Here's how the part is built. I have some questions about the finished solid (model axes, mm). A direction names the side the tool comes from. Round coordinates to 2 decimals unless told otherwise and drop trailing zeros. Write each loop counter-clockwise with the first axis right and the second up, starting at its lowest first coordinate (ties: lowest second). Pieces come first, ordered by that corner, then holes. Notation, with made-up numbers: (-36.5, -30) -> (6.5, -30) arc R32 ccw to (6.5, 4) -> close; hole circle Ø8 at (29, 48.5). An arc over 180 degrees is marked (long way). Answer as CSV lines item,"result".
```python
from build123d import *

# Parameters (mm, degrees)
SKETCH2_W           = 60
SKETCH2_H           = 60
BOSS_EXTRUDE1_DEPTH = 10
SKETCH3_R           = 2
CUT_EXTRUDE1_DEPTH  = 10
SKETCH5_R           = 2.7
CUT_EXTRUDE3_DEPTH  = 7
SKETCH6_R           = 0.5
CUT_EXTRUDE4_DEPTH  = 3
SKETCH7_R           = 6.75
CUT_EXTRUDE5_DEPTH  = 10


with BuildPart() as part:
    # Sketch2 → Boss-Extrude1 (new body)
    with BuildSketch(Plane(origin=(0, 0, 0), x_dir=(1, 0, 0), z_dir=(0, 1, 0))):
        Rectangle(SKETCH2_W, SKETCH2_H)
    extrude(amount=BOSS_EXTRUDE1_DEPTH)

    # Sketch3 → Cut-Extrude1 (cut)
    with BuildSketch(Plane(origin=(0, 10, 0), x_dir=(1, 0, 0), z_dir=(0, 1, 0))):
        with Locations((-26, 26)):
            Circle(SKETCH3_R)
        with Locations((-26, -26)):
            Circle(SKETCH3_R)
        with Locations((0, -26)):
            Circle(SKETCH3_R)
        with Locations((26, -26)):
            Circle(SKETCH3_R)
        with Locations((26, 26)):
            Circle(SKETCH3_R)
        with Locations((0, 26)):
            Circle(SKETCH3_R)
    extrude(amount=-CUT_EXTRUDE1_DEPTH, mode=Mode.SUBTRACT)

    # Sketch5 → Cut-Extrude3 (cut)
    with BuildSketch(Plane(origin=(0, 10, 0), x_dir=(1, 0, 0), z_dir=(0, 1, 0))):
        with Locations((12.5, 0)):
            Circle(SKETCH5_R)
        with Locations((-12.5, 0)):
            Circle(SKETCH5_R)
    extrude(amount=-CUT_EXTRUDE3_DEPTH, mode=Mode.SUBTRACT)

    # Sketch6 → Cut-Extrude4 (cut)
    with BuildSketch(Plane.XZ):
        with Locations((12.5, 0)):
            Circle(SKETCH6_R)
        with Locations((-12.5, 0)):
            Circle(SKETCH6_R)
    extrude(amount=-CUT_EXTRUDE4_DEPTH, mode=Mode.SUBTRACT)

    # Sketch7 → Cut-Extrude5 (cut)
    with BuildSketch(Plane(origin=(0, 10, 0), x_dir=(1, 0, 0), z_dir=(0, 1, 0))):
        Circle(SKETCH7_R)
    extrude(amount=-CUT_EXTRUDE5_DEPTH, mode=Mode.SUBTRACT)


solid = part.part
```
1. Suppose I cut it at B-B on z = 26. Please give me the cut outline in (x, y).
Numbers:
outline,"(-30, 0) -> (-28, 0) -> (-28, 10) -> (-30, 10) -> close; (-24, 0) -> (-2, 0) -> (-2, 10) -> (-24, 10) -> close; (2, 0) -> (24, 0) -> (24, 10) -> (2, 10) -> close; (28, 0) -> (30, 0) -> (30, 10) -> (28, 10) -> close"
2. If I drill on line 1 (Z direction, x = -26, y = 4); line 2 (X direction, y = 3, z = 26); line 3 (X direction, y = 3.25, z = 0), over which ranges is the centre line in solid material (lowest first)?
Numbers:
line 1,"z = -30 to -28, -24 to 24, 28 to 30"
line 2,"x = -30 to -28, -24 to -2, 2 to 24, 28 to 30"
line 3,"x = -30 to -15.2, -9.8 to -6.75, 6.75 to 9.8, 15.2 to 30"
3. If we mould it in two halves opening along Z, with no side actions, what happens to faces 1 (the face through (-7, 0, 0)), 2 (the face through (-26, 5, -24)), 3 (the face through (0, 5, 30))? For each: released by +Z, released by -Z, zero draft, split by the parting line, or undercut.
Numbers:
face 1,"zero draft"
face 2,"undercut"
face 3,"released by +Z"
4. Suppose I cut it at D-D on x = -26. Please give me the cut outline in (y, z), and give its area (3 significant figures).
Numbers:
outline,"(0, -30) -> (10, -30) -> (10, -28) -> (0, -28) -> close; (0, -24) -> (10, -24) -> (10, 24) -> (0, 24) -> close; (0, 28) -> (10, 28) -> (10, 30) -> (0, 30) -> close"
area,"520 mm^2"
5. For pin 1 Ø5 at (x, z) = (-12.5, 0) entering from +Y; pin 2 Ø5 at (x, z) = (-26, -26) entering from -Y, each with a flat end and sliding along its axis, tell me the tip position at first contact or that it passes through.
Numbers:
pin 1,"stops at y = 3"
pin 2,"stops at y = 0"
6. Suppose I cut it at A-A on x = 0. Please give me the cut outline in (y, z), and give its area (3 significant figures).
Numbers:
outline,"(0, -30) -> (10, -30) -> (10, -28) -> (0, -28) -> close; (0, -24) -> (10, -24) -> (10, -6.75) -> (0, -6.75) -> close; (0, 6.75) -> (10, 6.75) -> (10, 24) -> (0, 24) -> close; (0, 28) -> (10, 28) -> (10, 30) -> (0, 30) -> close"
area,"385 mm^2"
7. On a 3-axis mill with a long thin cutter (end or side, diameter ignored), from which of +Z, -Z, +X, -X, +Y, -Y can I reach the whole of each face in a straight line? I mean faces 4 (the face through (0, 5, -30)), 5 (the face through (-9.925, 6.549, -0.811)). Say none if no direction works.
Numbers:
face 4,"-Z, +X, -X, +Y, -Y"
face 5,"+Y"
8. Suppose I cut it at C-C on y = 6.75. Count the separate pieces of the cut face and the enclosed holes in it, and give its area (3 significant figures).
Numbers:
separate pieces,"1"
enclosed holes,"9"
area,"3,340 mm^2"
